```python
from build123d import *

# Parameters (mm, degrees)
BOSS_EXTRUDE1_DEPTH = 2.794
SKETCH2_W           = 1.5875
SKETCH2_H           = 6.35
CUT_EXTRUDE1_DEPTH  = 158.264546986
FILLET2_R           = 2.54
FILLET3_R           = 7.62
SKETCH4_R           = 2
SKETCH4_R_2         = 0.8
CUT_EXTRUDE2_DEPTH  = 157.484941985
CUT_EXTRUDE3_DEPTH  = 157.484941985
CUT_EXTRUDE4_DEPTH  = 157.484941985


with BuildPart() as part:
    # Sketch1 → Boss-Extrude1 (new body)
    with BuildSketch(Plane.ZY.offset(-5.715)):
        Polygon((-20.646158347, 31.796360983), (-20.646158347, 38.146360983), (-23.440158347, 38.146360983), (-23.440158347, 44.496360983), (-20.646158347, 44.496360983), (-20.646158347, 51.321360983), (11.831425782, 51.321360983), (64.730392893, 65.495596501), (64.730392893, 78.265338355), (9.737779753, 110.015338355), (22.437779753, 132.012383611), (33.106346702, 125.852883611), (26.756346702, 114.854360983), (60.411825944, 95.423360983), (66.761825944, 106.421883611), (77.430392893, 100.262383611), (82.628841653, 65.133860983), (82.628841653, 58.783860983), (85.422841653, 58.783860983), (85.422841653, 52.433860983), (82.628841653, 52.433860983), (82.628841653, 46.083860983), (41.353841653, 46.083860983), (41.353841653, 29.002360983), (35.003841653, 29.002360983), (35.003841653, 31.796360983), (-7.946158347, 31.796360983), (-7.946158347, 29.002360983), (-14.296158347, 29.002360983), (-14.296158347, 31.796360983), align=None)
    extrude(amount=BOSS_EXTRUDE1_DEPTH)

    # Sketch2 → Cut-Extrude1 (cut, through all)
    with BuildSketch(Plane.ZY.offset(-2.921)):
        with Locations((78.660091653, 52.433860983)):
            Rectangle(SKETCH2_W, SKETCH2_H)
    extrude(amount=-CUT_EXTRUDE1_DEPTH, mode=Mode.SUBTRACT)

    # Fillet2
    fillet2_edges = [part.edges().sort_by_distance(p)[0] for p in [
        (4.318, 132.012383611, 22.437779753),
        (4.318, 125.852883611, 33.106346702),
        (4.318, 114.854360983, 26.756346702),
        (4.318, 95.423360983, 60.411825944),
        (4.318, 106.421883611, 66.761825944),
        (4.318, 100.262383611, 77.430392893),
    ]]
    fillet(fillet2_edges, radius=FILLET2_R)

    # Fillet3
    fillet3_edges = [part.edges().sort_by_distance(p)[0] for p in [
        (4.318, 51.321360983, 11.831425782),
        (4.318, 65.495596501, 64.730392893),
        (4.318, 78.265338355, 64.730392893),
        (4.318, 110.015338355, 9.737779753),
    ]]
    fillet(fillet3_edges, radius=FILLET3_R)

    # Sketch4 → Cut-Extrude2 (cut, through all)
    with BuildSketch(Plane.ZY.offset(-2.921)):
        with Locations((-11.471158347, 43.146360983)):
            Circle(SKETCH4_R)
        with Locations((-6.971158347, 43.146360983)):
            Circle(SKETCH4_R_2)
        with Locations((-15.971158347, 43.146360983)):
            Circle(SKETCH4_R_2)
    extrude(amount=-CUT_EXTRUDE2_DEPTH, mode=Mode.SUBTRACT)

    # Sketch5 → Cut-Extrude3 (cut, through all)
    with BuildSketch(Plane.ZY.offset(-2.921)):
        Polygon((29.065685306, 41.392017329), (24.619477371, 36.945809394), (26.595133717, 34.970153047), (31.041341653, 39.416360983), align=None)
    extrude(amount=-CUT_EXTRUDE3_DEPTH, mode=Mode.SUBTRACT)

    # Sketch7 → Cut-Extrude4 (cut, through all)
    with BuildSketch(Plane.ZY.offset(-2.921)):
        Polygon((27.607085388, 129.027883611), (21.257085388, 118.029360983), (18.83741041, 119.426360983), (25.18741041, 130.424883611), align=None)
        Polygon((74.680762236, 101.849883611), (68.330762236, 90.851360983), (65.911087258, 92.248360983), (72.261087258, 103.246883611), align=None)
    extrude(amount=-CUT_EXTRUDE4_DEPTH, mode=Mode.SUBTRACT)


solid = part.part
```
The listing builds one solid part. Answer for the finished solid, in the listing's coordinates (mm). A direction names the side the tool comes from. Coordinates: 2 decimals unless noted, no trailing zeros. Write each loop counter-clockwise with the first axis right and the second up, starting at its lowest first coordinate (ties: lowest second). Pieces come first, ordered by that corner, then holes. Notation, with made-up numbers: (-34.5, 52) -> (-30.5, 52) arc R22 ccw to (-30.5, 74) -> close; hole circle Ø8 at (38, 74.5). An arc over 180 degrees is marked (long way). Write each question's results on one line, items separated by ' | '. Start each with the question number.
1) Straight lines are drawn through the part: probe 1 along Y at (x, z) = (4.1, -16); probe 2 along Y at (x, z) = (5.5, -11.5); probe 3 along Z at (x, y) = (4.1, 123.5). For each, find the intervals that lie inside material, in ascending order.
2) A tool of negligible diameter and unlimited length cuts with its end or side. For faces 1 (the flat face through (4, 73, 64.73)), 2 (the flat face through (4.3, 123.61, 24.48)), 3 (the flat face through (4, 30, -14.296)), 4 (the flat face through (4, 51.321, -5)), 5 (the flat face through (4, 38, 41.354)), from which of +Z, -Z, +X, -X, +Y, -Y can it reach the whole face along a straight path? Write none if from no direction.
3) For a pull along Y with two mould halves and no side action, classify faces 6 (the cylindrical face through (4.298, 44.833, -10.396)), 7 (the flat face through (4, 56, 85.423)), 8 (the flat face through (4.34, 100.88, 63.56)) as +Y half, -Y half, draft (parallel to the pull), parting line (faces both ways), or undercut.
4) Flat-ended cylindrical pins translate along their axes: pin 1 Ø0.8 at (x, y) = (4, 30) entering from -Z; pin 2 Ø0.5 at (x, z) = (4.5, 79) entering from -Y; pin 3 Ø0.8 at (x, z) = (4.5, -18) entering from -Y. Find the tip coordinate at first contact, or state that the pin passes through.
5) A cutting plane is placed at C-C (z = 3.5). Determine the outline of the cut face in (x, y) (3 decimals), then the cut area to 3 significant figures.
6) A cutting plane is placed at D-D (x = 4.15). Count the separate pieces of the cut face and the enclosed holes in it, then the cut area to 3 significant figures.
7) A cutting plane is placed at A-A (z = 63.5). Determine the outline of the cut face in (x, y) (3 decimals).
8) A cutting plane is placed at B-B (y = 121.5). Determine the outline of the cut face in (x, z) (3 decimals).
Values follow:
1) probe 1: 31.8 to 42.35, 43.95 to 51.32 | probe 2: 29 to 41.15, 45.15 to 51.32 | probe 3: 17.52 to 21.19, 24.42 to 31.75
2) face 1: -Z, +X, -X | face 2: +X, -X | face 3: -Z, +X, -X, -Y | face 4: -Z, +X, -X, +Y | face 5: +Z, +X, -X, -Y
3) face 6: undercut | face 7: draft | face 8: +Y half
4) pin 1: z = -14.3 | pin 2: y = 46.08 | pin 3: y = 31.8
5) outline: (2.921, 31.796) -> (5.715, 31.796) -> (5.715, 51.321) -> (2.921, 51.321) -> close | area: 54.6 mm²
6) separate pieces: 1 | enclosed holes: 5 | area: 3,520 mm²
7) outline: (2.921, 46.084) -> (5.715, 46.084) -> (5.715, 67.191) -> (2.921, 67.191) -> close; (2.921, 78.018) -> (5.715, 78.018) -> (5.715, 100.772) -> (2.921, 100.772) -> close
8) outline: (2.921, 16.368) -> (5.715, 16.368) -> (5.715, 20.035) -> (2.921, 20.035) -> close; (2.921, 23.261) -> (5.715, 23.261) -> (5.715, 30.593) -> (2.921, 30.593) -> close
